Check sheet for the drawn part. Datum: minimum x, y, z corner. Units: mm. Round coordinates to 2 decimals unless told otherwise and drop trailing zeros. Write each loop counter-clockwise with the first axis right and the second up, starting at its lowest first coordinate (ties: lowest second). Pieces come first, ordered by that corner, then holes. Notation, with made-up numbers: M -13,-24 L 24,-24 A15 cw 24,0 Z; hole C -9.5,-14 d7. An arc over 180 degrees is marked long. One line per item, written item: value. Start each with the question number.
Item 1: Thickness scan on probe 1 along Y at (x, z) = (6.35, 10.25); probe 2 along X at (y, z) = (8.89, 4.25); probe 3 along Y at (x, z) = (6.35, 5). Record the ranges inside material, lowest first. Write a range as from..to.
Item 2: Draft check along Z on the marked faces 1, 2, 3 and 4. Enter one of: +Z half, -Z half, draft (parallel to the pull), parting line (faces both ways), or undercut.
Item 3: Section check A-A, the plane x = 6.35. State how many separate pieces and enclosed holes the cut face has, then the cut area to 3 significant figures.
Item 4: Gauge pin test, flat end, axial feed: pin 1 (3 mm diameter, centred on x = 7, y = 13.5, fed in from -Z). Record the tip position at first contact, or that the pin passes through.
Item 5: Section check C-C, the plane y = 19.05. Record the cut outline in (x, z).
Item 6: Section check B-B, the plane z = 6.35. Record the cut outline in (x, y).
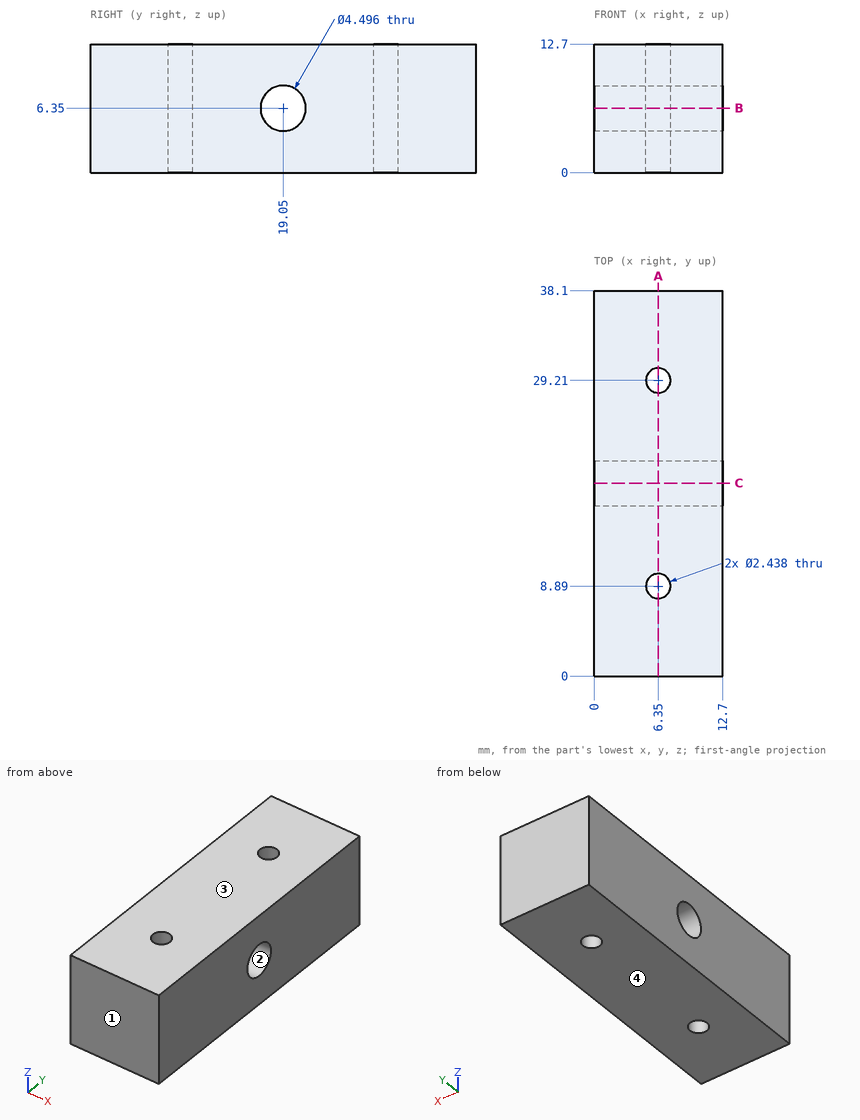
Response values:
1. probe 1: y = 0..7.67, 10.11..27.99, 30.43..38.1
1. probe 2: x = 0..5.13, 7.57..12.7
1. probe 3: y = 0..7.67, 10.11..17.25, 20.85..27.99, 30.43..38.1
2. face 1: draft
2. face 2: undercut
2. face 3: +Z half
2. face 4: -Z half
3. separate pieces: 3
3. enclosed holes: 1
3. area: 406 mm2
4. pin 1: stops at z = 0
5. outline: M 0,0 L 12.7,0 L 12.7,4.1 L 0,4.1 Z; M 0,8.6 L 12.7,8.6 L 12.7,12.7 L 0,12.7 Z
6. outline: M 0,0 L 12.7,0 L 12.7,16.8 L 0,16.8 Z; M 0,21.3 L 12.7,21.3 L 12.7,38.1 L 0,38.1 Z; hole C 6.35,8.89 d2.44; hole C 6.35,29.21 d2.44
